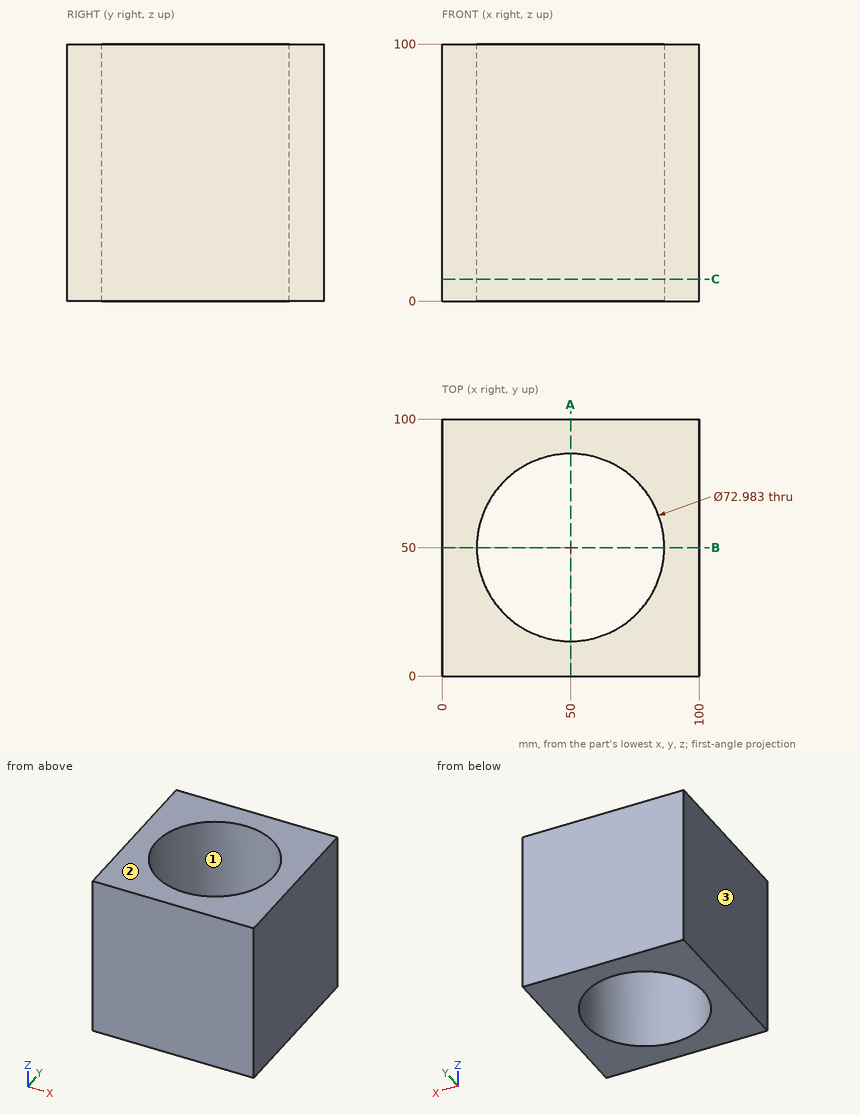
Geometry check sheet. Reference: drawing and pictorial views, mm from the part's lowest x, y, z. Round coordinates to 2 decimals unless told otherwise and drop trailing zeros. Write each loop counter-clockwise with the first axis right and the second up, starting at its lowest first coordinate (ties: lowest second). Pieces come first, ordered by that corner, then holes.
1. Section check A-A on x = 50. Enter the section's corners in (y, z).
2. Section check C-C on z = 8.5. Enter the section's corners in (x, y), plus the area to 3 significant figures.
3. Draft check along X on the marked faces 1, 2 and 3. Enter one of: +X half, -X half, draft (parallel to the pull), parting line (faces both ways), or undercut.
4. Scan lines: L1, parallel to Y at x = 50, z = 66; L2, parallel to X at y = 49, z = 79; L3, parallel to Y at x = 79, z = 67. Record each from-to range of solid material in increasing order.
Answer:
1. outline: (0, 0) - (13.51, 0) - (13.51, 100) - (0, 100) - close; (86.49, 0) - (100, 0) - (100, 100) - (86.49, 100) - close
2. outline: (0, 0) - (100, 0) - (100, 100) - (0, 100) - close; hole circle Ø72.98 at (50, 50)
2. area: 5,820 mm2
3. face 1: undercut
3. face 2: draft
3. face 3: -X half
4. L1: y = 0 to 13.51, 86.49 to 100
4. L2: x = 0 to 13.52, 86.48 to 100
4. L3: y = 0 to 27.85, 72.15 to 100
